For this review, take the finished solid that the model builds, in its own axes (mm). Round coordinates to 2 decimals unless told otherwise and drop trailing zeros. Write each loop counter-clockwise with the first axis right and the second up, starting at its lowest first coordinate (ties: lowest second). Pieces come first, ordered by that corner, then holes. Notation, with made-up numbers: (-21.75, 68.25) - (14.25, 68.25) arc R20 ccw to (14.25, 83.25) - close; hole circle Ø8 at (-1, 86). An arc over 180 degrees is marked (long way). One line per item, written item: value. Start each with the question number.
Q1. Add section C-C on z = 10. Write out the cut boundary in (x, y), and give its area (3 significant figures).
Q2. Mouldability with a two-part tool opening along X and no side actions: class faces 1 (the face through (-29.97, 1.32, 23.02)), 2 (the face through (-1, 45, 20)), 3 (the face through (-43.57, 0.56, 43.9)) as +X half, -X half, draft (parallel to the pull), parting line (faces both ways), or undercut.
Q3. For probe 1 along Y at (x, z) = (0, 19.5); probe 2 along Y at (x, z) = (19, 22); probe 3 along X at (y, z) = (-18.5, 3), list the stretches that pass through material, from the lowest coordinate up.
Q4. Add section A-A on y = 0. Write out the cut boundary in (x, z), and give its area (3 significant figures).
```python
from build123d import *

# Parameters (mm, degrees)
F0_W        = 90
F0_H        = 90
F1_DEPTH    = 45.4
F2_R        = 30
F3_DEPTH    = 45.401
F4_R        = 5
F5_T1_DEPTH = 52.9
F5_S5_W     = 5
F5_S5_H     = 5
F5_T6_DEPTH = 5


# Not quite as in the source:
# - a fillet or chamfer that OpenCascade refuses, or shapes differently, is made with other operations: its cross-section is extruded or revolved along the edge and cut away or added


with BuildPart() as f1:
    # F0 (on Top) → F1 (new body)
    with BuildSketch(Plane.XY):
        Rectangle(F0_W, F0_H)
    extrude(amount=F1_DEPTH)

    # F2 (on face) → F3 (cut, through all)
    with BuildSketch(Plane.XY.offset(45.4)):
        Circle(F2_R)
    extrude(amount=-F3_DEPTH, mode=Mode.SUBTRACT)

    # F4
    f4_edges = [f1.edges().sort_by_distance(p)[0] for p in [
        (-45, 45, 22.7),
        (-45, -45, 22.7),
        (45, 45, 22.7),
        (45, 0, 45.4),
        (-45, 0, 45.4),
        (0, 45, 45.4),
        (0, -45, 45.4),
    ]]
    fillet(f4_edges, radius=F4_R)

    # F5: fillet of radius 5 on 1 edges, made by hand

    # F5_s2 → F5_t1 (cut)
    with BuildSketch(Plane.XY.offset(-12.5)):
        with BuildLine():
            ThreePointArc((45, -40), (43.5355339059, -43.5355339059), (40, -45))
            Line((40, -45), (45, -45))
            Line((45, -45), (45, -40))
        make_face()
    extrude(amount=F5_T1_DEPTH, mode=Mode.SUBTRACT)


with BuildPart() as f5_tool4:
    # F5_s5 → F5_t6 (new body)
    with BuildSketch(Plane.YZ.offset(40)):
        with Locations((-42.5, 42.9)):
            Rectangle(F5_S5_W, F5_S5_H)
    extrude(amount=F5_T6_DEPTH)

    # F5_s7 → F5_t8 (revolve, cut)
    with BuildSketch(Plane(origin=(40, -40, 40.4), x_dir=(0, 0.7071067812, -0.7071067812), z_dir=(0, -0.7071067812, -0.7071067812))):
        with BuildLine():
            ThreePointArc((0, -5), (5, 0), (0, 5))
            Line((0, 5), (0, -5))
        make_face()
    revolve(axis=Axis((40, -40, 40.4), (1, 0, 0)), mode=Mode.SUBTRACT)


with BuildPart() as f1_1:
    add(f1.part)

    # F5_t3: cut F5_tool4
    add(f5_tool4.part, mode=Mode.SUBTRACT)


solid = f1_1.part
```
Result set:
1. outline: (-45, -40) arc R5 ccw to (-40, -45) - (40, -45) arc R5 ccw to (45, -40) - (45, 40) arc R5 ccw to (40, 45) - (-40, 45) arc R5 ccw to (-45, 40) - close; hole circle Ø60 at (0, 0)
1. area: 5,250 mm^2
2. face 1: undercut
2. face 2: draft
2. face 3: -X half
3. probe 1: y = -45 to -30, 30 to 45
3. probe 2: y = -45 to -23.22, 23.22 to 45
3. probe 3: x = -45 to -23.62, 23.62 to 45
4. outline: (-45, 0) - (-30, 0) - (-30, 45.4) - (-40, 45.4) arc R5 ccw to (-45, 40.4) - close; (30, 0) - (45, 0) - (45, 40.4) arc R5 ccw to (40, 45.4) - (30, 45.4) - close
4. area: 1,350 mm^2
